Geometry: see drawing. Coordinates: mm, zero at the bounding-box minimum. A direction names the side the tool comes from. Round coordinates to 2 decimals unless told otherwise and drop trailing zeros. Order: outer loops, then holes, each group sorted by start corner. A loop starts at its lowest first (then second) coordinate and runs counter-clockwise, first axis right, second up. Notation, with made-up numbers: (-38.5, 77) -> (-12.5, 77) arc R24 ccw to (-12.5, 110) -> close; hole circle Ø11 at (22.5, 28.5). An arc over 180 degrees is marked (long way). Use a Markdown table: item, result.
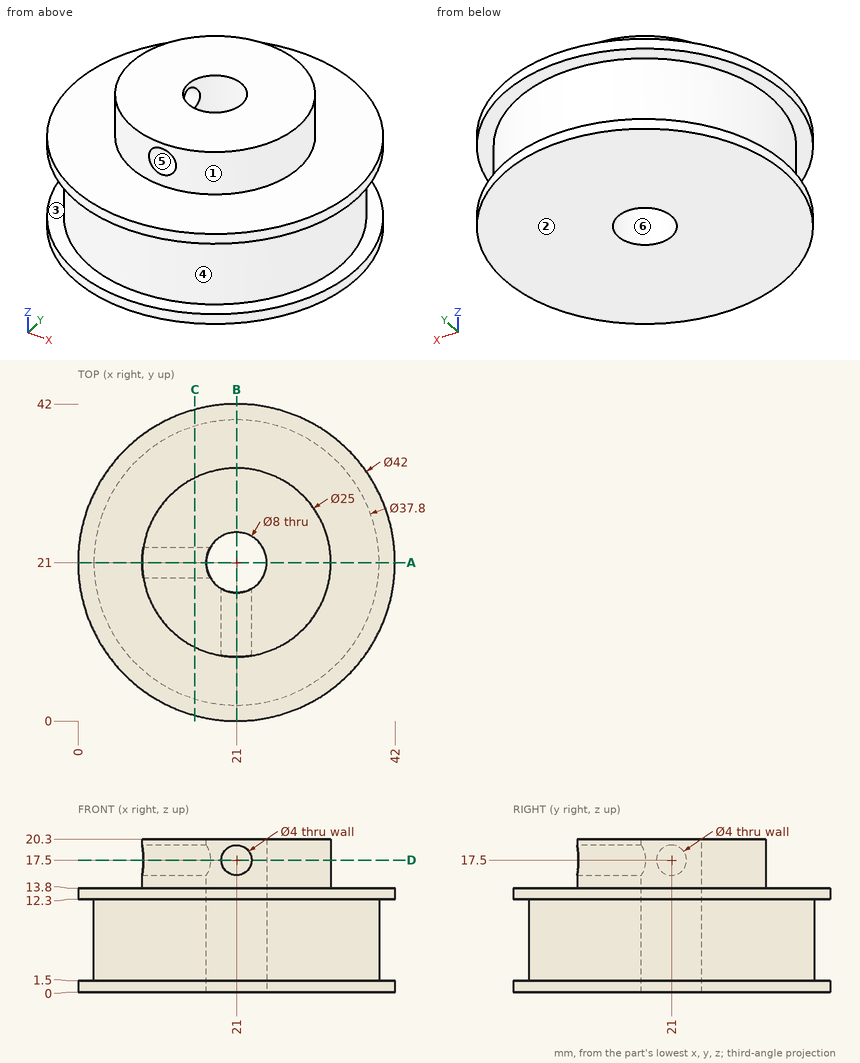
1) Cut plane D-D on z = 17.5. Return loops of the section in (x, y), and give its area (3 significant figures).
Answer key:
| item | result |
|---|---|
| outline | (8.66, 19) arc R12.5 ccw to (19, 8.66) -> (19, 17.54) arc R4 cw to (17.54, 19) -> close; (8.66, 23) -> (17.54, 23) arc R4 cw (long way) to (23, 17.54) -> (23, 8.66) arc R12.5 ccw (long way) to start |
| area | 372 mm^2 |
2) Cut plane A-A on y = 21. Return loops of the section in (x, z), and give its area (3 significant figures).
Answer key:
| item | result |
|---|---|
| outline | (0, 0) -> (17, 0) -> (17, 15.5) -> (8.5, 15.5) -> (8.5, 13.8) -> (0, 13.8) -> (0, 12.3) -> (2.1, 12.3) -> (2.1, 1.5) -> (0, 1.5) -> close; (8.5, 19.5) -> (17, 19.5) -> (17, 20.3) -> (8.5, 20.3) -> close; (25, 0) -> (42, 0) -> (42, 1.5) -> (39.9, 1.5) -> (39.9, 12.3) -> (42, 12.3) -> (42, 13.8) -> (33.5, 13.8) -> (33.5, 20.3) -> (25, 20.3) -> close |
| area | 500 mm^2 |
3) Contact query for flat-ended pins moving along their axis: P1, Ø1, axis at x = 28, y = 33, coming from the +Z side; P2, Ø6, axis at x = 10, z = 15, coming from the +Y side; P3, Ø10, axis at y = 25.5, z = 16.5, coming from the -X side; P4, Ø5, axis at x = 21, y = 21, coming from the +Z side. Output: stop coordinate, or through.
Answer key:
| item | result |
|---|---|
| P1 | stops at z = 13.8 |
| P2 | stops at y = 40.31 |
| P3 | stops at x = 0 |
| P4 | passes through |
4) Draft query along Y for the marked faces 4, 5 and 6. Return one class per face: released by +Y, released by -Y, zero draft, split by the parting line, or undercut.
Answer key:
| item | result |
|---|---|
| face 4 | split by the parting line |
| face 5 | zero draft |
| face 6 | undercut |
5) Cut plane C-C on x = 15.5. Return loops of the section in (y, z).
Answer key:
| item | result |
|---|---|
| outline | (0.73, 0) -> (41.27, 0) -> (41.27, 1.5) -> (39.08, 1.5) -> (39.08, 12.3) -> (41.27, 12.3) -> (41.27, 13.8) -> (32.22, 13.8) -> (32.22, 20.3) -> (9.78, 20.3) -> (9.78, 13.8) -> (0.73, 13.8) -> (0.73, 12.3) -> (2.92, 12.3) -> (2.92, 1.5) -> (0.73, 1.5) -> close; hole circle Ø4 at (21, 17.5) |
6) Ray query, probe 1 along Z at (x, y) = (21, 12); probe 2 along X at (y, z) = (21, 15); probe 3 along Y at (x, z) = (21, 10.5). Return the intervals inside material, ascending.
Answer key:
| item | result |
|---|---|
| probe 1 | z = 0 to 15.5, 19.5 to 20.3 |
| probe 2 | x = 8.5 to 17, 25 to 33.5 |
| probe 3 | y = 2.1 to 17, 25 to 39.9 |
7) Set-up query: the marked faces 1, 2 and 3. Return all of +Z, -Z, +X, -X, +Y, -Y with unobstructed straight access to the full face (end or side cutting, diameter ignored); none if empty.
Answer key:
| item | result |
|---|---|
| face 1 | +Z |
| face 2 | -Z, +X, -X, +Y, -Y |
| face 3 | none |
